Could you check a few things on this model? Use its own coordinates, in mm. A direction names the side the tool comes from. Coordinates: 2 decimals unless noted, no trailing zeros. Order: outer loops, then holes, each group sorted by start corner. A loop starts at its lowest first (then second) coordinate and runs counter-clockwise, first axis right, second up. Notation, with made-up numbers: (31.5, -28.5) - (59.5, -28.5) arc R21 cw to (59.5, 9.5) - close; hole circle Ø5 at (77, 39.5). An arc over 180 degrees is marked (long way). Answer as a JSON object with one key per item and string values. Group by question number.
(1) Please list where these lines run through material, in increasing order: probe 1 along X at (y, z) = (1.6, -52); probe 2 along Z at (x, y) = (15.5, 3.05); probe 3 along X at (y, z) = (0.7, 3).
(2) Imagine slicing it at B-B, the plane y = 3.05. Give the number of separate pieces and of enclosed holes in the cut face, and give its area (3 significant figures).
(3) Imagine slicing it at C-C, the plane x = -82. Write out the boundary of the cut face in (y, z), and give its area (3 significant figures).
(4) We'd pull the mould along X, two halves only. Please class faces 4 (the flat face through (-102, 2, -76)), 5 (the cylindrical face through (-23.57, 2.54, 24.6)), 6 (the flat face through (114, 2, 61)): pulls with the +X half, pulls with the -X half, needs draft (parallel to the pull), parting line crosses it, or undercut.
(5) Imagine slicing it at A-A, the plane z = -11. Write out the boundary of the cut face in (x, y).
(6) Will these pins go through, and if not, where does the flat tip stop? P1, Ø1.5, axis at x = -19, y = 2.5, coming from the -Z side; P2, Ø2, axis at x = -21.5, y = 3, coming from the +Z side.
(7) Which directions (+Z, -Z, +X, -X, +Y, -Y) give clear straight access to the entire face, cutting with the end or side of a thin tool? Please do faces 1 (the flat face through (-26, 2, 73)), 2 (the flat face through (29, 3, 0)), 3 (the flat face through (76, 2, -73)).
from build123d import *

# Parameters (mm, degrees)
SKETCH1_W           = 3
SKETCH1_H           = 30.4
SKETCH1_W_2         = 18.8
SKETCH1_H_2         = 4.8
BOSS_EXTRUDE1_DEPTH = 5
CUT_EXTRUDE1_DEPTH  = 138.102151697


with BuildPart() as part:
    # Sketch1 → Boss-Extrude1 (new body)
    with BuildSketch(Plane(origin=(0, 0, 0), x_dir=(1, 0, 0), z_dir=(0, 1, 0))):
        Polygon((-114, 0), (-114, 15.2), (-111, 15.2), (-111, 45.6), (-114, 45.6), (-114, 76), (-88.666666667, 76), (-88.666666667, 73), (-63.333333333, 73), (-63.333333333, 76), (-38, 76), (-38, 73), (-12.666666667, 73), (-12.666666667, 76), (0, 76), (0, 0), (-33, 0), (-33, 15.2), (-38, 15.2), (-38, 0), align=None)
        with Locations((-39.5, 40.8)):
            Rectangle(SKETCH1_W, SKETCH1_H, mode=Mode.SUBTRACT)
        with Locations((-19, 32.5)):
            Rectangle(SKETCH1_W_2, SKETCH1_H_2, mode=Mode.SUBTRACT)
    boss_extrude1 = extrude(amount=BOSS_EXTRUDE1_DEPTH)

    # Mirror1: Boss-Extrude1 across plane
    add(boss_extrude1.mirror(Plane(origin=(-114, 5, 0), x_dir=(1, 0, 0), z_dir=(0, 0, -1))))

    # Mirror6: part across plane


with BuildPart() as part_1:
    add(part.part)
    add(part.part.mirror(Plane(origin=(0, 5, 0), x_dir=(0, 0, 1), z_dir=(-1, 0, 0))))

    # Sketch2 → Cut-Extrude1 (cut, through all)
    with BuildSketch(Plane(origin=(0, 5, 0), x_dir=(1, 0, 0), z_dir=(0, 1, 0))):
        with BuildLine():
            Line((24, 26.1), (-20, 26.1))
            ThreePointArc((-20, 26.1), (-23.535533906, 24.635533906), (-25, 21.1))
            Line((-25, 21.1), (-25, -21.1))
            ThreePointArc((-25, -21.1), (-23.535533906, -24.635533906), (-20, -26.1))
            Line((-20, -26.1), (24, -26.1))
            ThreePointArc((24, -26.1), (27.535533906, -24.635533906), (29, -21.1))
            Line((29, -21.1), (29, 21.1))
            ThreePointArc((29, 21.1), (27.535533906, 24.635533906), (24, 26.1))
        make_face()
    extrude(amount=-CUT_EXTRUDE1_DEPTH, mode=Mode.SUBTRACT)


solid = part_1.part
Result set:
{
 "1": {"probe 1": "x = -114 to -41, -38 to 38, 41 to 114", "probe 2": "z = -73 to -34.9, -30.1 to -26.1, 26.1 to 30.1, 34.9 to 73", "probe 3": "x = -114 to -38, -33 to -25, 29 to 33, 38 to 114"},
 "2": {"separate pieces": "1", "enclosed holes": "11", "area": "29,900 mm^2"},
 "3": {"outline": "(0, -73) - (5, -73) - (5, 73) - (0, 73) - close", "area": "730 mm^2"},
 "4": {"face 4": "needs draft", "face 5": "undercut", "face 6": "pulls with the +X half"},
 "5": {"outline": "(-114, 0) - (-38, 0) - (-38, 5) - (-114, 5) - close; (-33, 0) - (-25, 0) - (-25, 5) - (-33, 5) - close; (29, 0) - (33, 0) - (33, 5) - (29, 5) - close; (38, 0) - (114, 0) - (114, 5) - (38, 5) - close"},
 "6": {"P1": "stops at z = -73", "P2": "stops at z = 73"},
 "7": {"face 1": "+Z, +Y, -Y", "face 2": "+Y, -Y", "face 3": "-Z, +Y, -Y"}
}
